from build123d import *

# Parameters (mm, degrees)
ESBO_O1_W                = 150
ESBO_O1_H                = 150
ESBO_O1_R                = 1.5
ESBO_O1_W_2              = 41.5
ESBO_O1_H_2              = 21
RESSALTO_EXTRUS_O1_DEPTH = 4


with BuildPart() as part:
    # Esboço1 → Ressalto-extrusão1 (new body)
    with BuildSketch(Plane.XY):
        Rectangle(ESBO_O1_W, ESBO_O1_H)
        with Locations((-66.55, 60.5)):
            Circle(ESBO_O1_R, mode=Mode.SUBTRACT)
        with Locations((-66.55, 50.5)):
            Circle(ESBO_O1_R, mode=Mode.SUBTRACT)
        with Locations(Location((-17.95, 60.5, 0), (0, 0, 180))):
            Circle(ESBO_O1_R, mode=Mode.SUBTRACT)
        with Locations(Location((-17.95, 50.5, 0), (0, 0, 180))):
            Circle(ESBO_O1_R, mode=Mode.SUBTRACT)
        with Locations((17.95, 50.5)):
            Circle(ESBO_O1_R, mode=Mode.SUBTRACT)
        with Locations((17.95, 60.5)):
            Circle(ESBO_O1_R, mode=Mode.SUBTRACT)
        with Locations(Location((66.55, 50.5, 0), (0, 0, 180))):
            Circle(ESBO_O1_R, mode=Mode.SUBTRACT)
        with Locations(Location((66.55, 60.5, 0), (0, 0, 180))):
            Circle(ESBO_O1_R, mode=Mode.SUBTRACT)
        with Locations((66.55, -60.5)):
            Circle(ESBO_O1_R, mode=Mode.SUBTRACT)
        with Locations((66.55, -50.5)):
            Circle(ESBO_O1_R, mode=Mode.SUBTRACT)
        with Locations(Location((17.95, -60.5, 0), (0, 0, 180))):
            Circle(ESBO_O1_R, mode=Mode.SUBTRACT)
        with Locations(Location((17.95, -50.5, 0), (0, 0, 180))):
            Circle(ESBO_O1_R, mode=Mode.SUBTRACT)
        with Locations((-17.95, -50.5)):
            Circle(ESBO_O1_R, mode=Mode.SUBTRACT)
        with Locations((-17.95, -60.5)):
            Circle(ESBO_O1_R, mode=Mode.SUBTRACT)
        with Locations(Location((-66.55, -50.5, 0), (0, 0, 180))):
            Circle(ESBO_O1_R, mode=Mode.SUBTRACT)
        with Locations(Location((-66.55, -60.5, 0), (0, 0, 180))):
            Circle(ESBO_O1_R, mode=Mode.SUBTRACT)
        with Locations((-42.25, 55.5)):
            Rectangle(ESBO_O1_W_2, ESBO_O1_H_2, mode=Mode.SUBTRACT)
        with Locations((42.25, 55.5)):
            Rectangle(ESBO_O1_W_2, ESBO_O1_H_2, mode=Mode.SUBTRACT)
        with Locations((42.25, -55.5)):
            Rectangle(ESBO_O1_W_2, ESBO_O1_H_2, mode=Mode.SUBTRACT)
        with Locations((-42.25, -55.5)):
            Rectangle(ESBO_O1_W_2, ESBO_O1_H_2, mode=Mode.SUBTRACT)
    extrude(amount=RESSALTO_EXTRUS_O1_DEPTH)


solid = part.part
Could you check a few things on this model? Use its own coordinates, in mm. A direction names the side the tool comes from. Round coordinates to 2 decimals unless told otherwise and drop trailing zeros. Order: outer loops, then holes, each group sorted by start corner. A loop starts at its lowest first (then second) coordinate and runs counter-clockwise, first axis right, second up.
Q1. Imagine slicing it at B-B, the plane y = 64. List the corners of the cut face in (x, z) for me, then the cut area to 3 significant figures.
Geometry says:
outline: (-75, 0) - (-63, 0) - (-63, 4) - (-75, 4) - close; (-21.5, 0) - (21.5, 0) - (21.5, 4) - (-21.5, 4) - close; (63, 0) - (75, 0) - (75, 4) - (63, 4) - close
area: 268 mm2
Q2. Which directions (+Z, -Z, +X, -X, +Y, -Y) give clear straight access to the entire face, cutting with the end or side of a thin tool? Please do faces 1 (the face through (-63, -56, 2)), 2 (the face through (75, -1, 2)).
Geometry says:
face 1: +Z, -Z
face 2: +Z, -Z, +X, +Y, -Y
Q3. I'm going to push a flat-ended pin straight in: P1, Ø2.5, axis at x = 17.95, y = 50.5, coming from the -Z side. Where does the tip first touch, or does it pass through?
Geometry says:
P1: passes through
Q4. Imagine slicing it at A-A, the plane x = -57. List the corners of the cut face in (y, z) for me.
Geometry says:
outline: (-75, 0) - (-66, 0) - (-66, 4) - (-75, 4) - close; (-45, 0) - (45, 0) - (45, 4) - (-45, 4) - close; (66, 0) - (75, 0) - (75, 4) - (66, 4) - close
Q5. Please list where these lines run through material, in increasing order: probe 1 along Y at (x, z) = (-55, 2.05); probe 2 along Y at (x, z) = (17.95, 2.1); probe 3 along X at (y, z) = (54.5, 2.8).
Geometry says:
probe 1: y = -75 to -66, -45 to 45, 66 to 75
probe 2: y = -75 to -62, -59 to -52, -49 to 49, 52 to 59, 62 to 75
probe 3: x = -75 to -63, -21.5 to 21.5, 63 to 75
Q6. Imagine slicing it at C-C, the plane z = 2.2. State how many separate pieces and enclosed holes the cut face has, then the cut area to 3 significant figures.
Geometry says:
separate pieces: 1
enclosed holes: 20
area: 18,900 mm2
Q7. Thinking about a two-plate mould opening in Y: for faces 3 (the face through (-1, -75, 2)), 4 (the face through (-1, 75, 2)), 5 (the face through (-21.5, -56, 2)), which applies, released by +Y, released by -Y, zero draft, split by the parting line, or undercut?
Geometry says:
face 3: released by -Y
face 4: released by +Y
face 5: undercut
